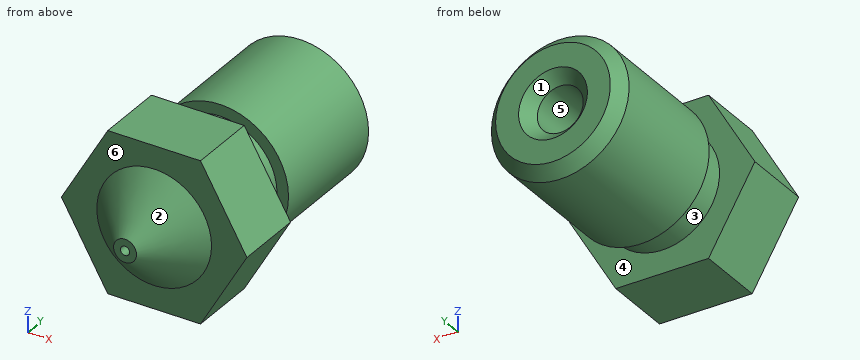
```python
from build123d import *

# Parameters (mm, degrees)
BOSS_EXTRUDE1_DEPTH = 3
CHAMFER1_SIZE       = 0.5


with BuildPart() as part:
    # Sketch1 → Boss-Extrude1 (new body)
    with BuildSketch(Plane.XZ):
        Polygon((-2.020725942, 3.5), (-4.041451884, 0), (-2.020725942, -3.5), (2.020725942, -3.5), (4.041451884, 0), (2.020725942, 3.5), align=None)
    extrude(amount=-BOSS_EXTRUDE1_DEPTH)

    # Sketch2 → Revolve1 (revolve)
    with BuildSketch(Plane(origin=(0, 0, 0), x_dir=(-1, 0, 0), z_dir=(0, 0, -1))):
        Polygon((-2.5, 3), (0, 3), (0, 10.5), (-3, 10.5), (-3, 4.5), (-2.5, 4.5), align=None)
    revolve(axis=Axis((0, 3, 0), (0, 1, 0)))

    # Sketch3 → Revolve2 (revolve)
    with BuildSketch(Plane.XY):
        Polygon((2.5, 0), (0, 0), (0, -2), (0.5, -2), align=None)
    revolve(axis=Axis((0, 0, 0), (0, -1, 0)))

    # Sketch4 → Cut-Revolve1 (revolve, cut)
    with BuildSketch(Plane(origin=(0, 0, 0), x_dir=(-1, 0, 0), z_dir=(0, 0, -1))):
        Polygon((-0.2, -2), (0, -2), (0, 10.5), (-1, 10.5), (-1, 0), (-0.75, -0.227272727), (-0.75, -0.7), (-0.2, -1.2), align=None)
    revolve(axis=Axis((0, -2, 0), (0, 1, 0)), mode=Mode.SUBTRACT)

    # Chamfer1
    chamfer1_edges = [part.edges().sort_by_distance(p)[0] for p in [
        (-3, 10.5, 0),
        (-1, 10.5, 0),
    ]]
    chamfer(chamfer1_edges, length=CHAMFER1_SIZE)


solid = part.part
```
Part model, mm, in its own coordinate system. Face numbers are marked on the shaded views. A direction names the side the tool comes from. Give positions to 0.01 mm unless a question says otherwise; leave off trailing zeros. Order: outer loops, then holes, each group sorted by start corner. A loop starts at its lowest first (then second) coordinate and runs counter-clockwise, first axis right, second up. Notation, with made-up numbers: (73.5, 9) - (123.5, 9) arc R21 cw to (123.5, 39) - close; hole circle Ø11 at (44, -38). An arc over 180 degrees is marked (long way). Use one line per item in the form item = value.
Item 1: Slice it at A-A on y = 2.75. Give the cut face in (x, z), and give its area (3 significant figures).
Solution:
outline = (-4.04, 0) - (-2.02, -3.5) - (2.02, -3.5) - (4.04, 0) - (2.02, 3.5) - (-2.02, 3.5) - close; hole circle Ø2 at (0, 0)
area = 39.3 mm2
Item 2: Probe probe 1 along X at (y, z) = (5, 0); probe 2 along X at (y, z) = (3.25, 0); probe 3 along Z at (x, y) = (0, 2.75). List the from-to ranges inside material, lowest first. Write a range as from..to.
Solution:
probe_1 = -3..-1, 1..3
probe_2 = -2.5..-1, 1..2.5
probe_3 = -3.5..-1, 1..3.5
Item 3: Two-plate mould, pull along Y, no slides. Class the marked faces 1, 2 and 3: released by +Y, released by -Y, zero draft, split by the parting line, or undercut.
Solution:
face_1 = released by +Y
face_2 = released by -Y
face_3 = undercut
Item 4: Slice it at C-C on y = 8. Give the cut face in (x, z).
Solution:
outline = circle Ø6 at (0, 0); hole circle Ø2 at (0, 0)
Item 5: Which spindle directions (+Z, -Z, +X, -X, +Y, -Y) get a long thin tool onto all of the face, cutting with end or side? Do the marked faces 4, 5 and 6. Say none if no direction does.
Solution:
face_4 = none
face_5 = +Y
face_6 = -Y
Item 6: Pin check, flat tips, straight feed: pin 1 Ø1.4 at (x, z) = (0, 0) entering from +Y; pin 2 Ø3.5 at (x, z) = (0.5, -0.5) entering from -Y; pin 3 Ø2.5 at (x, z) = (0, 0) entering from +Y; pin 4 Ø1.5 at (y, z) = (3, -2.5) entering from +X. Stop position of each tip, or through.
Solution:
pin_1 = -0.75
pin_2 = -2
pin_3 = 10.25
pin_4 = 3.03
